Here's how the part is built. I have some questions about the finished solid (model axes, mm). A direction names the side the tool comes from. Round coordinates to 2 decimals unless told otherwise and drop trailing zeros. Order: outer loops, then holes, each group sorted by start corner. A loop starts at its lowest first (then second) coordinate and runs counter-clockwise, first axis right, second up.
```python
from build123d import *

# Parameters (mm, degrees)
SKETCH042_R   = 1.6
SKETCH042_R_2 = 1.5
SKETCH042_R_3 = 2
SKETCH042_W   = 15
SKETCH042_H   = 6.2
SKETCH042_W_2 = 16
SKETCH042_W_3 = 6.1
SKETCH042_H_2 = 16
PAD_DEPTH     = 6


with BuildPart() as part:
    # Sketch042 → Pad (new body)
    with BuildSketch(Plane.XY):
        with BuildLine():
            ThreePointArc((-10, -104.5), (0, -114.5), (10, -104.5))
            ThreePointArc((107, 82.3), (35.695621, 0.741674), (10, -104.5))
            Line((107, 82.3), (107, 94.817542))
            ThreePointArc((108.875, 102.079385), (107.476312, 98.567542), (107, 94.817542))
            ThreePointArc((108.875, 102.079385), (108.035534, 108.035534), (102.079385, 108.875))
            ThreePointArc((94.817542, 107), (98.567542, 107.476312), (102.079385, 108.875))
            Line((94.817542, 107), (52.717063, 107))
            ThreePointArc((-52.717063, 107), (0, 93.4), (52.717063, 107))
            Line((-52.717063, 107), (-94.817542, 107))
            ThreePointArc((-102.079385, 108.875), (-98.567542, 107.476312), (-94.817542, 107))
            ThreePointArc((-102.079385, 108.875), (-108.035534, 108.035534), (-108.875, 102.079385))
            ThreePointArc((-107, 94.817542), (-107.476312, 98.567542), (-108.875, 102.079385))
            Line((-107, 94.817542), (-107, 82.3))
            ThreePointArc((-10, -104.5), (-35.695621, 0.741674), (-107, 82.3))
        make_face()
        with Locations((34, 43.8)):
            Circle(SKETCH042_R, mode=Mode.SUBTRACT)
        with Locations((9.53018, -64.149856)):
            Circle(SKETCH042_R_2, mode=Mode.SUBTRACT)
        with Locations((-104.5, 104.5)):
            Circle(SKETCH042_R_2, mode=Mode.SUBTRACT)
        with Locations((28, 85.4)):
            Circle(SKETCH042_R_3, mode=Mode.SUBTRACT)
        with Locations((0, -104.5)):
            Circle(SKETCH042_R_2, mode=Mode.SUBTRACT)
        with Locations((-28, 85.4)):
            Circle(SKETCH042_R_3, mode=Mode.SUBTRACT)
        with Locations((-34, 43.8)):
            Circle(SKETCH042_R, mode=Mode.SUBTRACT)
        with Locations((0, 54.4)):
            Circle(SKETCH042_R_3, mode=Mode.SUBTRACT)
        with Locations((0, -45.6)):
            Circle(SKETCH042_R_3, mode=Mode.SUBTRACT)
        with Locations((104.5, 104.5)):
            Circle(SKETCH042_R_2, mode=Mode.SUBTRACT)
        with Locations((37.131304, 11.683608)):
            Circle(SKETCH042_R_2, mode=Mode.SUBTRACT)
        with Locations((89.004449, 73.503615)):
            Circle(SKETCH042_R_2, mode=Mode.SUBTRACT)
        with Locations((0, 85.4)):
            Rectangle(SKETCH042_W, SKETCH042_H, mode=Mode.SUBTRACT)
        with Locations((74, 85.4)):
            Rectangle(SKETCH042_W_2, SKETCH042_H, mode=Mode.SUBTRACT)
        with Locations((0, -84.6)):
            Rectangle(SKETCH042_W_3, SKETCH042_H_2, mode=Mode.SUBTRACT)
        with Locations((-74, 85.4)):
            Rectangle(SKETCH042_W_2, SKETCH042_H, mode=Mode.SUBTRACT)
    extrude(amount=PAD_DEPTH)


solid = part.part
```
1. I need wall thicknesses on probe 1 along X at (y, z) = (104.5, 2.65); probe 2 along X at (y, z) = (89.5, 4.7); probe 3 along Y at (x, z) = (-104.5, 4.25). Which ranges of each line are inside material? Lowest first, please.
Evaluation:
probe 1: x = -109.5 to -106, -103 to -47.92, 47.92 to 103, 106 to 109.5
probe 2: x = -107 to 107
probe 3: y = 80.52 to 103, 106 to 109.5
2. If we section it at A-A, the plane y = -52.5: Write out the boundary of the cut face in (x, z).
Evaluation:
outline: (-16, 0) - (16, 0) - (16, 6) - (-16, 6) - close
3. If we section it at C-C, the plane x = -23: Write out the boundary of the cut face in (y, z).
Evaluation:
outline: (-28.55, 0) - (95.85, 0) - (95.85, 6) - (-28.55, 6) - close
4. On a 3-axis mill with a long thin cutter (end or side, diameter ignored), from which of +Z, -Z, +X, -X, +Y, -Y can I reach the whole of each face in a straight line? I mean faces 5 (the flat face through (0, -92.6, 3)), 6 (the flat face through (-73, 107, 3)), 7 (the flat face through (107, 88, 3)), 8 (the cylindrical face through (-34.995, -0.62, 2.958)). Say none if no direction works.
Evaluation:
face 5: +Z, -Z
face 6: +Z, -Z, +Y
face 7: +Z, -Z, +X, -Y
face 8: +Z, -Z, -X, -Y
5. I'm going to push flat-ended pins straight in: P1, Ø3, axis at x = 55, z = 5, coming from the +Y side; P2, Ø3, axis at x = -72, z = 1.5, coming from the -Y side; P3, Ø3, axis at y = 9, z = 1, coming from the +X side. Where does each tip first touch, or does it pass through?
Evaluation:
P1: stops at y = 107
P2: stops at y = 50.33
P3: stops at x = 41.07
6. If we section it at B-B, the plane z = 4.5: State how many separate pieces and enclosed holes the cut face has, and give its area (3 significant figures).
Evaluation:
separate pieces: 1
enclosed holes: 16
area: 18,600 mm2
7. If we mould it in two halves opening along Y, with no side actions, what happens to faces 1 (the flat face through (-107, 89, 3)), 2 (the flat face through (-7.5, 85, 3)), 3 (the flat face through (-82, 85, 3)), 4 (the flat face through (74, 107, 3))? For each: released by +Y, released by -Y, zero draft, split by the parting line, or undercut.
Evaluation:
face 1: zero draft
face 2: undercut
face 3: undercut
face 4: released by +Y
